Could you check a few things on this model? Use its own coordinates, in mm. Face numbers are marked on the shaded views. A direction names the side the tool comes from. Coordinates: 2 decimals unless noted, no trailing zeros. Write each loop counter-clockwise with the first axis right and the second up, starting at its lowest first coordinate (ties: lowest second). Pieces come first, ordered by that corner, then holes. Notation, with made-up numbers: M -31,-21 L -19,-21 A18 ccw -19,10 Z; hole C 0.25,79.25 d10. An arc over 180 degrees is marked long. Answer as CSV lines item,"result". Start each with the question number.
Item 1: Suppose I cut it at A-A, the plane x = 24. Write out the boundary of the cut face in (y, z), and give its area (3 significant figures).
Item 2: Suppose I cut it at D-D, the plane z = 11.75. Write out the boundary of the cut face in (x, y), and give its area (3 significant figures).
Item 3: Suppose I cut it at B-B, the plane z = 6. Write out the boundary of the cut face in (x, y), and give its area (3 significant figures).
Item 4: Suppose I cut it at C-C, the plane y = -5. Write out the boundary of the cut face in (x, z).
Item 5: If I drill on line 1 along Z through (x, y) = (13, -7.5); line 2 along Y through (x, z) = (4.5, 6.25); line 3 along X through (y, z) = (-7.5, 10), over which ranges is the centre line in solid material (lowest first)? Write a range as [from, to].
Item 6: On a 3-axis mill with a long thin cutter (end or side, diameter ignored), from which of +Z, -Z, +X, -X, +Y, -Y can I reach the whole of each face in a straight line? I mean the marked faces 1 and 2. Say none if no direction works.
Item 7: We'd pull the mould along Y, two halves only. Please class the marked faces 3, 4 and 5: +Y half, -Y half, draft (parallel to the pull), parting line (faces both ways), or undercut.
Item 8: I'm going to push flat-ended pins straight in: P1, Ø1.7, axis at x = -1.5, z = 3, coming from the +Y side; P2, Ø1.5, axis at y = 1, z = 11, coming from the -X side; P3, Ø4, axis at y = -14.5, z = 10, coming from the +X side; P4, Ø0.7, axis at y = -17, z = 3, coming from the +X side. Where does each tip first touch, or does it pass through?
Autodesk Inventor part; units mm, degrees
ref_plane "YZ Plane" through (0, 0, 0) normal (1, 0, 0) x (0, 1, 0)
ref_plane "XZ Plane" through (0, 0, 0) normal (0, 1, 0) x (-1, 0, 0)
ref_plane "XY Plane" through (0, 0, 0) normal (0, 0, 1) x (1, 0, 0)
sketch "Эскиз1" plane through (0, 0, 0) normal (0, 0, 1) x (1, 0, 0)
  line L0 (-29, 18) -> (29, 18)
  line L1 (30, 17) -> (30, -17)
  line L2 (29, -18) -> (-29, -18)
  line L3 (-30, -17) -> (-30, 17)
  arc A0 (-29, 18) -> (-30, 17) centre (-29, 17) ccw
  arc A1 (-30, -17) -> (-29, -18) centre (-29, -17) ccw
  arc A2 (29, -18) -> (30, -17) centre (29, -17) ccw
  arc A3 (30, 17) -> (29, 18) centre (29, 17) ccw
  point P0 (0, 0)
  point P1 (-30, 18)
  point P2 (30, 18)
  point P3 (-30, -18)
  dimension "d0" = 60
  dimension "d1" = 36
  dimension "d2" = 18
  dimension "d3" = 30
  dimension "d4" = 1
extrude "Выдавливание1" add sketch "Эскиз1" along normal blind 4
sketch "Эскиз3" plane through (0, 0, 4) normal (0, 0, 1) x (1, 0, 0)
  line L0 (-29, 18) -> (29, 18)
  line L1 (30, 17) -> (30, -17)
  line L2 (29, -18) -> (-29, -18)
  line L3 (-30, -17) -> (-30, 17)
  line L4 (30, -17) -> (30, 17)
  line L5 (-29, -18) -> (29, -18)
  line L6 (-30, 17) -> (-30, -17)
  line L7 (29, 18) -> (-29, 18)
  arc A0 (-29, 18) -> (-30, 17) centre (-29, 17) ccw
  arc A1 (-30, -17) -> (-29, -18) centre (-29, -17) ccw
  arc A2 (29, -18) -> (30, -17) centre (29, -17) ccw
  arc A3 (30, 17) -> (29, 18) centre (29, 17) ccw
  point P0 (0, 0)
  dimension "d7" = 0
  dimension "d8" = 0
  dimension "d9" = 0
  dimension "d10" = 0
  dimension "d11" = 1
extrude "Выдавливание2" add sketch "Эскиз3" along normal blind 10 draft -3
sketch "Эскиз4" plane through (0, 0, 0) normal (0, 0, -1) x (-1, 0, 0)
  line L0 (-27.5, 15.5) -> (27.5, 15.5)
  line L1 (27.5, 15.5) -> (27.5, -15.5)
  line L2 (27.5, -15.5) -> (-27.5, -15.5)
  line L3 (-27.5, -15.5) -> (-27.5, 15.5)
  point P0 (0, 0)
  dimension "d14" = 15.5
  dimension "d15" = 31
  dimension "d16" = 27.5
  dimension "d17" = 55
extrude "Выдавливание3" cut sketch "Эскиз4" against normal blind 13 draft -3
sketch "Эскиз5" plane through (0, 0, 0) normal (0, 0, -1) x (-1, 0, 0)
  line L0 (-28.5, 16.5) -> (28.5, 16.5)
  line L1 (28.5, 16.5) -> (28.5, -16.5)
  line L2 (28.5, -16.5) -> (-28.5, -16.5)
  line L3 (-28.5, -16.5) -> (-28.5, 16.5)
  line L4 (-29, 18) -> (29, 18)
  line L5 (-30, -17) -> (-30, 17)
  line L6 (29, -18) -> (-29, -18)
  line L7 (30, 17) -> (30, -17)
  line L8 (-29, 18) -> (29, 18)
  line L9 (30, 17) -> (30, -17)
  line L10 (29, -18) -> (-29, -18)
  line L11 (-30, -17) -> (-30, 17)
  arc A0 (-29, 18) -> (-30, 17) centre (-29, 17) ccw
  arc A1 (-30, -17) -> (-29, -18) centre (-29, -17) ccw
  arc A2 (29, -18) -> (30, -17) centre (29, -17) ccw
  arc A3 (30, 17) -> (29, 18) centre (29, 17) ccw
  point P0 (0, 0)
  point P1 (29, 18)
  dimension "d20" = 1.5
  dimension "d21" = 1.5
  dimension "d22" = 1.5
  dimension "d23" = 1.5
  dimension "d24" = 0
  dimension "d25" = 0
  dimension "d26" = 0
  dimension "d27" = 0
  dimension "d28" = 1
extrude "Выдавливание4" cut sketch "Эскиз5" against normal blind 4
fillet "Сопряжение1" radius 1 8 edges at (-29.3365, -17.3365, 14) (-29.4759, 0, 14) (-29.3365, 17.3365, 14) (0, 17.4759, 14) (29.3365, 17.3365, 14) (29.4759, 0, 14) (29.3365, -17.3365, 14) (0, -17.4759, 14)
sketch "Эскиз6" plane through (-28.5, -16.5, 0) normal (0, -1, 0) x (1, 0, 0)
  line L0 (0, 4) -> (23.5, 4)
  line L1 (23.5, 4) -> (23.5, 0)
  line L2 (23.5, 0) -> (0, 0)
  line L3 (0, 0) -> (0, 4)
  line L4 (33.5, 4) -> (57, 4)
  line L5 (57, 4) -> (57, 0)
  line L6 (57, 0) -> (33.5, 0)
  line L7 (33.5, 0) -> (33.5, 4)
  line L8 (-0.5, 4) -> (57.5, 4)
  line L9 (57, 0) -> (0, 0)
  line L10 (0, 0) -> (0, 4)
  line L11 (57, 0) -> (57, 4)
  point P0 (28.5, 0)
  dimension "d32" = 0
  dimension "d33" = 0
  dimension "d34" = 0
  dimension "d35" = 23.5
  dimension "d36" = 0
  dimension "d37" = 23.5
extrude "Выдавливание5" cut sketch "Эскиз6" against normal through all contours L0 L1 L2 L3 | L4 L5 L6 L7
sketch "Эскиз8" plane through (-5, -16.5, 0) normal (0, -1, 0) x (1, 0, 0)
  line L0 (0, 1.9) -> (10, 1.9)
  line L1 (10, 1.9) -> (10, 0)
  line L2 (10, 0) -> (0, 0)
  line L3 (0, 0) -> (0, 1.9)
  line L4 (0, 4) -> (0, 0)
  line L5 (10, 0) -> (0, 0)
  line L6 (10, 0) -> (10, 4)
  point P0 (5, 0)
  dimension "d43" = 0
  dimension "d44" = 0
  dimension "d45" = 0
  dimension "d46" = 1.9
extrude "Выдавливание6" add sketch "Эскиз8" along normal blind 1
sketch "Эскиз9" plane through (-5, 16.5, 0) normal (0, 1, 0) x (1, 0, 0)
  line L0 (10, -1.9) -> (0, -1.9)
  line L1 (0, -1.9) -> (0, 0)
  line L2 (0, 0) -> (10, 0)
  line L3 (10, 0) -> (10, -1.9)
  line L4 (0, 0) -> (10, 0)
  line L5 (10, -4) -> (10, 0)
  line L6 (0, 0) -> (0, -4)
  point P0 (5, 0)
  dimension "d49" = 0
  dimension "d50" = 0
  dimension "d51" = 0
  dimension "d52" = 1.9
extrude "Выдавливание7" add sketch "Эскиз9" along normal blind 1
sketch "Эскиз10" plane through (5, -16.5, 4) normal (1, 0, 0) x (0, 0, -1)
  line L0 (4, 0) -> (2.1, -1)
  line L1 (4, 34) -> (2.1, 34)
  line L2 (2.1, 34) -> (4, 33)
  line L3 (2.1, 34) -> (4, 34)
  line L4 (4, 33) -> (4, 34)
  line L5 (2.1, -1) -> (4, -1)
  line L6 (2.1, -1) -> (4, -1)
  line L7 (4, -1) -> (4, 0)
  line L8 (4, -1) -> (4, 1)
  point P0 (4, 16.5)
extrude "Выдавливание8" cut sketch "Эскиз10" against normal through all
properties part number "case_up" material "Пластик АБС"
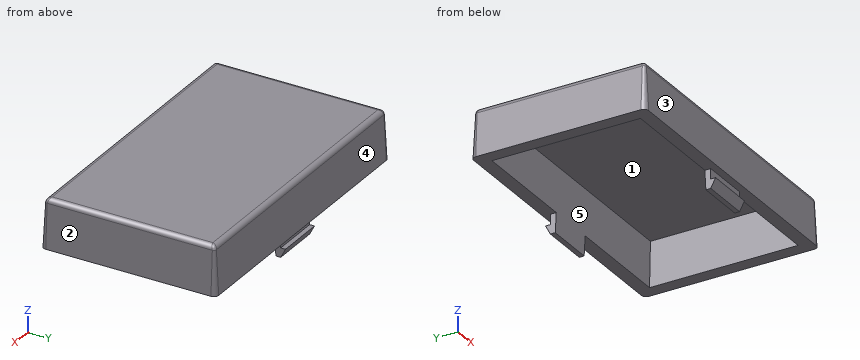
Ans:
1,outline,"M -18,4 L -15.29,4 L -14.82,13 L 14.82,13 L 15.29,4 L 18,4 L 17.53,13.05 A1 ccw 16.53,14 L -16.53,14 A1 ccw -17.53,13.05 Z"
1,area,"83.4 mm^2"
2,outline,"M -29.59,-17 A0.59 ccw -29,-17.59 L 29,-17.59 A0.59 ccw 29.59,-17 L 29.59,17 A0.59 ccw 29,17.59 L -29,17.59 A0.59 ccw -29.59,17 Z; hole M -26.88,-14.88 L 26.88,-14.88 L 26.88,14.88 L -26.88,14.88 Z"
2,area,"482 mm^2"
3,outline,"M -29.9,-17 A0.9 ccw -29,-17.9 L 29,-17.9 A0.9 ccw 29.9,-17 L 29.9,17 A0.9 ccw 29,17.9 L -29,17.9 A0.9 ccw -29.9,17 Z; hole M -27.19,-15.19 L 27.19,-15.19 L 27.19,15.19 L -27.19,15.19 Z"
3,area,"488 mm^2"
4,outline,"M -30,4 L -27.29,4 L -26.82,13 L 26.82,13 L 27.29,4 L 30,4 L 29.53,13.05 A1 ccw 28.53,14 L -28.53,14 A1 ccw -29.53,13.05 Z"
5,line 1,"z = [13, 14]"
5,line 2,"y = [-17.88, -15.17], [15.17, 17.88]"
5,line 3,"x = [-29.69, -26.98], [26.98, 29.69]"
6,face 1,"-Z"
6,face 2,"+Z, +X, +Y, -Y"
7,face 3,"-Y half"
7,face 4,"+Y half"
7,face 5,"undercut"
8,P1,"stops at y = 16.5"
8,P2,"stops at x = -29.67"
8,P3,"stops at x = 29.79"
8,P4,"passes through"
